Part model, mm, in its own coordinate system. A direction names the side the tool comes from. Give positions to 0.01 mm unless a question says otherwise; leave off trailing zeros. Order: outer loops, then holes, each group sorted by start corner. A loop starts at its lowest first (then second) coordinate and runs counter-clockwise, first axis right, second up.
1. Slice it at A-A on y = 30. List the corners of the cut face in (x, z), and give its area (3 significant figures).
2. Mould opens along X. For faces 4 (the cylindrical face through (-3, 4, -37)), 5 (the flat face through (0, -7, -12)), 6 (the cylindrical face through (0.74, 26.68, 5.42)) say: +X half, -X half, draft (parallel to the pull), parting line (faces both ways), or undercut.
3. Slice it at C-C on x = 29. List the corners of the cut face in (y, z), and give its area (3 significant figures).
4. Drop flat-ended pins along their axis: pin 1 Ø10 at (x, y) = (-2, -1) entering from -Z; pin 2 Ø1.3 at (y, z) = (-4, -37.5) entering from +X; pin 3 Ø8 at (y, z) = (8, -12) entering from +X; pin 4 Ø1 at (x, y) = (-7, 19.5) entering from -Z. Give the stop position or say it passes through.
5. Probe line 1 (Z direction, x = 29, y = 5); line 2 (Z direction, x = -5, y = 1); line 3 (Y direction, x = 30, z = 6). List the from-to ranges inside material, lowest first.
6. Slice it at D-D on y = -25. List the corners of the cut face in (x, z), and give its area (3 significant figures).
7. Slice it at B-B on z = -39.5. List the corners of the cut face in (x, y), and give its area (3 significant figures).
8. Which spindle directions (+Z, -Z, +X, -X, +Y, -Y) get a long thin tool onto all of the face, cutting with end or side? Do faces 1 (the cylindrical face through (-30.594, -27.813, 8.535)), 2 (the flat face through (0, -3.2, -37)), 3 (the cylindrical face through (11.99, 0.53, -0.49)). Say none if no direction does.
from build123d import *

# Parameters (mm, degrees)
SKETCH1_R                                     = 37.5
BOSS_EXTRUDE1_DEPTH                           = 11
TAP_DRILL_FOR_M8_TAP1_D                       = 6.8
TAP_DRILL_FOR_M8_TAP1_DEPTH                   = 23
TAP_DRILL_FOR_M8_TAP1_TIP                     = 2.042926105
SKETCH6_R                                     = 12
BOSS_EXTRU_1_DEPTH                            = 1
SKETCH5_R                                     = 10
BOSS_EXTRU_2_DEPTH                            = 11
ESQUISSE1_R                                   = 6
BOSS_EXTRU_3_DEPTH                            = 14
ESQUISSE4_R                                   = 5
BOSS_EXTRU_4_DEPTH                            = 22
TROU_POUR_TARAUDAGE_POUR_TROU_TARAUD_M6_D     = 5
TROU_POUR_TARAUDAGE_POUR_TROU_TARAUD_M6_DEPTH = 23
TROU_POUR_TARAUDAGE_POUR_TROU_TARAUD_M6_TIP   = 1.502151548
ENL_V_START                                   = -3.2
ENL_V_MAT_EXTRU_1_DEPTH                       = 10
BOSS_EXTRU_5_DEPTH                            = 5
TROU_POUR_TARAUDAGE_POUR_TROU_TARAUD_M8_D     = 6.8
TROU_POUR_TARAUDAGE_POUR_TROU_TARAUD_M8_DEPTH = 8
TROU_POUR_TARAUDAGE_POUR_TROU_TARAUD_M8_TIP   = 2.042926105


with BuildPart() as part:
    # Sketch1 → Boss-Extrude1 (new body)
    with BuildSketch(Plane.XY):
        Circle(SKETCH1_R)
    extrude(amount=BOSS_EXTRUDE1_DEPTH)

    # Tap Drill for M8 Tap1
    with Locations(Plane.XY.offset(11)):
        with Locations((-30, 0), (0, 30), (30, 0), (0, -30)):
            Hole(TAP_DRILL_FOR_M8_TAP1_D / 2, depth=TAP_DRILL_FOR_M8_TAP1_DEPTH)
            with Locations((0, 0, -(TAP_DRILL_FOR_M8_TAP1_DEPTH + TAP_DRILL_FOR_M8_TAP1_TIP / 2))):  # 118° drill point
                Cone(0, TAP_DRILL_FOR_M8_TAP1_D / 2, TAP_DRILL_FOR_M8_TAP1_TIP, mode=Mode.SUBTRACT)

    # Sketch6 → Boss.-Extru.1 (add)
    with BuildSketch(Plane(origin=(0, 0, 0), x_dir=(-1, 0, 0), z_dir=(0, 0, -1))):
        Circle(SKETCH6_R)
    extrude(amount=BOSS_EXTRU_1_DEPTH)

    # Sketch5 → Boss.-Extru.2 (add)
    with BuildSketch(Plane(origin=(0, 0, -1), x_dir=(-1, 0, 0), z_dir=(0, 0, -1))):
        Circle(SKETCH5_R)
    extrude(amount=BOSS_EXTRU_2_DEPTH)

    # Esquisse1 → Boss.-Extru.3 (add)
    with BuildSketch(Plane(origin=(0, 0, -12), x_dir=(-1, 0, 0), z_dir=(0, 0, -1))):
        Circle(ESQUISSE1_R)
    extrude(amount=BOSS_EXTRU_3_DEPTH)

    # Esquisse4 → Boss.-Extru.4 (add)
    with BuildSketch(Plane(origin=(0, 0, -26), x_dir=(-1, 0, 0), z_dir=(0, 0, -1))):
        Circle(ESQUISSE4_R)
    extrude(amount=BOSS_EXTRU_4_DEPTH)

    # Trou pour taraudage pour trou taraudé M61
    with Locations(Plane(origin=(0, 0, -48), x_dir=(-1, 0, 0), z_dir=(0, 0, -1))):
        with Locations((0, 0)):
            Hole(TROU_POUR_TARAUDAGE_POUR_TROU_TARAUD_M6_D / 2, depth=TROU_POUR_TARAUDAGE_POUR_TROU_TARAUD_M6_DEPTH)
            with Locations((0, 0, -(TROU_POUR_TARAUDAGE_POUR_TROU_TARAUD_M6_DEPTH + TROU_POUR_TARAUDAGE_POUR_TROU_TARAUD_M6_TIP / 2))):  # 118° drill point
                Cone(0, TROU_POUR_TARAUDAGE_POUR_TROU_TARAUD_M6_D / 2, TROU_POUR_TARAUDAGE_POUR_TROU_TARAUD_M6_TIP, mode=Mode.SUBTRACT)

    # Esquisse5 → Enlèv. mat.-Extru.1 (cut)
    with BuildSketch(Plane(origin=(0, 0, 0), x_dir=(1, 0, 0), z_dir=(0, 1, 0)).offset(ENL_V_START)):
        with BuildLine():
            Line((-1.5, 27.923988696), (-1.5, 48))
            ThreePointArc((-1.5, 48), (0, 49.5), (1.5, 48))
            Line((1.5, 48), (1.5, 27.923988696))
            ThreePointArc((1.5, 27.923988696), (0, 26.423988696), (-1.5, 27.923988696))
        make_face()
    extrude(amount=-ENL_V_MAT_EXTRU_1_DEPTH, mode=Mode.SUBTRACT)

    # Esquisse6 → Boss.-Extru.5 (add)
    with BuildSketch(Plane.XY.offset(11)):
        with BuildLine():
            ThreePointArc((-46.154891817, -18.608064174), (-49.363448016, -28.5), (-39.192502198, -30.667276735))
            ThreePointArc((-39.192502198, -30.667276735), (-30.463205965, -27.811629704), (-21.705713829, -30.579600834))
            ThreePointArc((-21.705713829, -30.579600834), (-32.475952642, -18.75), (-37.335568074, -3.507899166))
            ThreePointArc((-37.335568074, -3.507899166), (-39.317180827, -12.476095394), (-46.154891817, -18.608064174))
        make_face()
    extrude(amount=-BOSS_EXTRU_5_DEPTH)

    # Trou pour taraudage pour trou taraudé M81
    with Locations(Plane.XY.offset(11)):
        with Locations((-43.301270189, -25)):
            Hole(TROU_POUR_TARAUDAGE_POUR_TROU_TARAUD_M8_D / 2, depth=TROU_POUR_TARAUDAGE_POUR_TROU_TARAUD_M8_DEPTH)
            with Locations((0, 0, -(TROU_POUR_TARAUDAGE_POUR_TROU_TARAUD_M8_DEPTH + TROU_POUR_TARAUDAGE_POUR_TROU_TARAUD_M8_TIP / 2))):  # 118° drill point
                Cone(0, TROU_POUR_TARAUDAGE_POUR_TROU_TARAUD_M8_D / 2, TROU_POUR_TARAUDAGE_POUR_TROU_TARAUD_M8_TIP, mode=Mode.SUBTRACT)


solid = part.part
Data:
1. outline: (-22.5, 0) - (-3.4, 0) - (-3.4, 11) - (-22.5, 11) - close; (3.4, 0) - (22.5, 0) - (22.5, 11) - (3.4, 11) - close
1. area: 420 mm2
2. face 4: parting line
2. face 5: draft
2. face 6: undercut
3. outline: (-23.77, 0) - (-3.25, 0) - (-3.25, 11) - (-23.77, 11) - close; (3.25, 0) - (23.77, 0) - (23.77, 11) - (3.25, 11) - close
3. area: 452 mm2
4. pin 1: stops at z = -48
4. pin 2: stops at x = 3.71
4. pin 3: stops at x = 9.17
4. pin 4: stops at z = 0
5. line 1: z = 0 to 11
5. line 2: z = -26 to 11
5. line 3: y = -22.5 to -3.4, 3.4 to 22.5
6. outline: (-50.3, 6) - (-46.7, 6) - (-46.7, 11) - (-50.3, 11) - close; (-39.9, 6) - (-27.95, 6) - (-27.95, 0) - (27.95, 0) - (27.95, 11) - (-39.9, 11) - close
6. area: 693 mm2
7. outline: (-1.5, -4.77) - (-1.5, -3.2) - (1.5, -3.2) - (1.5, -4.77) arc R5 ccw (long way) to start; hole circle Ø5 at (0, 0)
7. area: 53.7 mm2
8. face 1: +Z, -Z, -Y
8. face 2: -Z, -Y
8. face 3: -Z
